Verification items for this drawing (mm, ordinates from the low corner). A direction names the side the tool comes from. Give positions to 0.01 mm unless a question says otherwise; leave off trailing zeros. Loops run counter-clockwise (first coordinate to the right, second up) from the corner with the lowest first, then second, coordinate; pieces in that order, holes last. Notation, with made-up numbers: (-31, 9) -> (8, 9) arc R5 ccw to (8, 14) -> close; hole circle Ø1 at (-34.5, 83). An arc over 180 degrees is marked (long way). Answer in a Markdown table with one row per item. Add a question column.
Q1. Section check D-D on x = 33. Enter the section's corners in (y, z), and give its area (3 significant figures).
Q2. Release check for a two-part mould opening along X. For the marked faces 3, 4 and 5 record: pulls with the +X half, pulls with the -X half, needs draft (parallel to the pull), parting line crosses it, or undercut.
Q3. Set-up check for the marked faces 1 and 2: record each of +Z, -Z, +X, -X, +Y, -Y from which the full face is reachable in a straight line by a thin tool's end or side.
Q4. Section check A-A on z = 9.75. Enter the section's corners in (x, y).
Q5. Section check B-B on y = 8.5. Enter the section's corners in (x, z).
Q6. Gauge pin test, flat ends, axial feed: P1, Ø1.6, axis at x = 14.5, y = 1.5, coming from the +Z side; P2, Ø3, axis at x = 10.5, y = 23.5, coming from the +Z side; P3, Ø2, axis at x = 11, z = 7.5, coming from the +Y side. Record the tip position at first contact, or that the pin passes through.
Q7. Material ranges on probe 1 along X at (y, z) = (15.5, 13.75); probe 2 along X at (y, z) = (26, 9); probe 3 along Z at (x, y) = (14.5, 15.5), recorded low to high.
Q8. Section check C-C on z = 7. Enter the section's corners in (x, y).
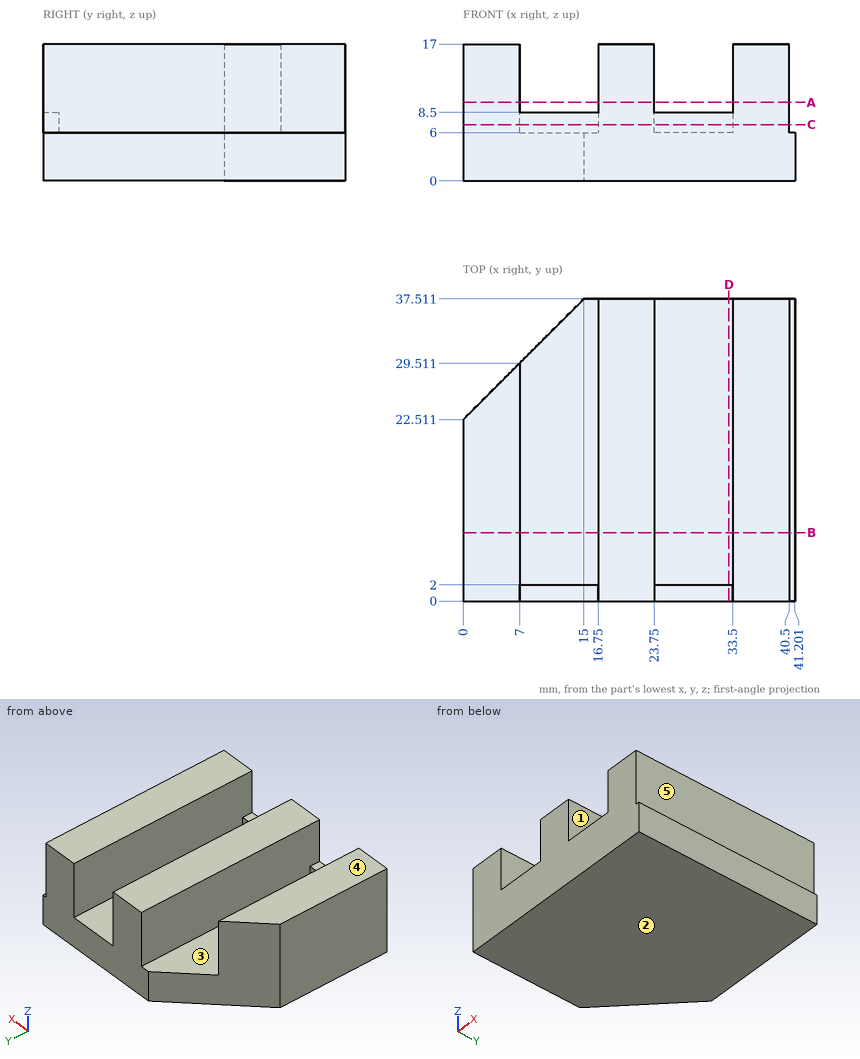
Taken from the geometry:
| question | item | result |
|---|---|---|
| 1 | outline | (0, 0) -> (37.51, 0) -> (37.51, 6) -> (2, 6) -> (2, 8.5) -> (0, 8.5) -> close |
| 1 | area | 230 mm² |
| 2 | face 3 | undercut |
| 2 | face 4 | needs draft |
| 2 | face 5 | pulls with the +X half |
| 3 | face 1 | +Z, +Y |
| 3 | face 2 | -Z, +X, -X, +Y, -Y |
| 4 | outline | (0, 0) -> (7, 0) -> (7, 29.51) -> (0, 22.51) -> close; (16.75, 0) -> (23.75, 0) -> (23.75, 37.51) -> (16.75, 37.51) -> close; (33.5, 0) -> (40.5, 0) -> (40.5, 37.51) -> (33.5, 37.51) -> close |
| 5 | outline | (0, 0) -> (41.2, 0) -> (41.2, 6) -> (40.5, 6) -> (40.5, 17) -> (33.5, 17) -> (33.5, 6) -> (23.75, 6) -> (23.75, 17) -> (16.75, 17) -> (16.75, 6) -> (7, 6) -> (7, 17) -> (0, 17) -> close |
| 6 | P1 | stops at z = 8.5 |
| 6 | P2 | stops at z = 6 |
| 6 | P3 | stops at y = 2 |
| 7 | probe 1 | x = 0 to 7, 16.75 to 23.75, 33.5 to 40.5 |
| 7 | probe 2 | x = 3.49 to 7, 16.75 to 23.75, 33.5 to 40.5 |
| 7 | probe 3 | z = 0 to 6 |
| 8 | outline | (0, 0) -> (40.5, 0) -> (40.5, 37.51) -> (33.5, 37.51) -> (33.5, 2) -> (23.75, 2) -> (23.75, 37.51) -> (16.75, 37.51) -> (16.75, 2) -> (7, 2) -> (7, 29.51) -> (0, 22.51) -> close |
